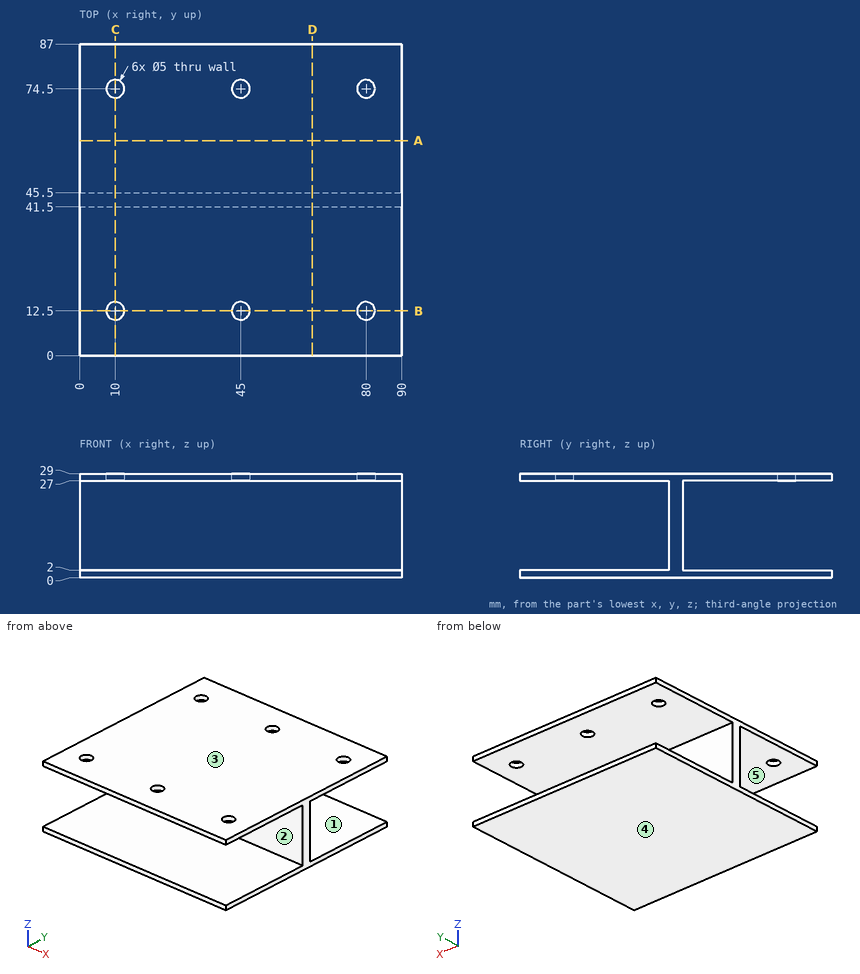
Part print with two shaded views. Sizes in mm from the minimum x, y, z corner. A direction names the side the tool comes from. Round coordinates to 2 decimals unless told otherwise and drop trailing zeros. Loops run counter-clockwise (first coordinate to the right, second up) from the corner with the lowest first, then second, coordinate; pieces in that order, holes last. Notation, with made-up numbers: (53.25, -35) - (109.25, -35) arc R8 ccw to (109.25, -26) - close; hole circle Ø4 at (46.25, 1). An arc over 180 degrees is marked (long way). Put each result on its own line as item: value.
1. Slice it at B-B on y = 12.5. List the corners of the cut face in (x, z), and give its area (3 significant figures).
Geometry check:
outline: (0, 0) - (90, 0) - (90, 2) - (0, 2) - close; (0, 27) - (7.5, 27) - (7.5, 29) - (0, 29) - close; (12.5, 27) - (42.5, 27) - (42.5, 29) - (12.5, 29) - close; (47.5, 27) - (77.5, 27) - (77.5, 29) - (47.5, 29) - close; (82.5, 27) - (90, 27) - (90, 29) - (82.5, 29) - close
area: 330 mm²
2. Slice it at C-C on x = 10. List the corners of the cut face in (y, z), and give its area (3 significant figures).
Geometry check:
outline: (0, 0) - (87, 0) - (87, 2) - (45.5, 2) - (45.5, 27) - (72, 27) - (72, 29) - (15, 29) - (15, 27) - (41.5, 27) - (41.5, 2) - (0, 2) - close; (0, 27) - (10, 27) - (10, 29) - (0, 29) - close; (77, 27) - (87, 27) - (87, 29) - (77, 29) - close
area: 428 mm²
3. Pin check, flat tip, straight feed: P1, Ø3, axis at x = 28.5, z = 23.5, coming from the +Y side. Stop position of the tip, or through.
Geometry check:
P1: y = 45.5
4. Slice it at D-D on x = 65. List the corners of the cut face in (y, z).
Geometry check:
outline: (0, 0) - (87, 0) - (87, 2) - (45.5, 2) - (45.5, 27) - (87, 27) - (87, 29) - (0, 29) - (0, 27) - (41.5, 27) - (41.5, 2) - (0, 2) - close
5. Two-plate mould, pull along Z, no slides. Class the marked faces 3, 4 and 5: released by +Z, released by -Z, zero draft, split by the parting line, or undercut.
Geometry check:
face 3: released by +Z
face 4: released by -Z
face 5: undercut
6. 3-axis set-ups, long thin cutter, end or side, ignore diameter. For the marked faces 1 and 2: which of +Z, -Z, +X, -X, +Y, -Y reach the whole face in a straight line?
Geometry check:
face 1: +X, -X, +Y
face 2: +X, -X, -Y
7. Wall check: line 1 (Y direction, x = 45, z = 27.85); line 2 (X direction, y = 74.5, z = 27.5); line 3 (Z direction, x = 52, y = 40.5). Give the ranges that are in metal, low to high.
Geometry check:
line 1: 0 to 10, 15 to 72, 77 to 87
line 2: 0 to 7.5, 12.5 to 42.5, 47.5 to 77.5, 82.5 to 90
line 3: 0 to 2, 27 to 29
8. Slice it at A-A on y = 60. List the corners of the cut face in (x, z), and give its area (3 significant figures).
Geometry check:
outline: (0, 0) - (90, 0) - (90, 2) - (0, 2) - close; (0, 27) - (90, 27) - (90, 29) - (0, 29) - close
area: 360 mm²
